from build123d import *

# Parameters (mm, degrees)
SKETCH1_W           = 20
SKETCH1_H           = 40
BOSS_EXTRUDE1_DEPTH = 20
CUT_EXTRUDE1_DEPTH  = 2


with BuildPart() as part:
    # Sketch1 → Boss-Extrude1 (new body)
    with BuildSketch(Plane(origin=(0, 0, 0), x_dir=(1, 0, 0), z_dir=(0, 1, 0))):
        Rectangle(SKETCH1_W, SKETCH1_H)
    extrude(amount=BOSS_EXTRUDE1_DEPTH)

    # Sketch2 → Cut-Extrude1 (cut)
    with BuildSketch(Plane(origin=(0, 20, 0), x_dir=(1, 0, 0), z_dir=(0, 1, 0))):
        Polygon((-3.5, -6.730769231), (-3.5, -6.416666667), (-2.064102564, -6.416666667), (-2.064102564, -4.621794872), (-3.5, -4.621794872), (-3.5, -4.307692308), (0, -4.307692308), (0, -4.621794872), (-1.705128205, -4.621794872), (-1.705128205, -6.416666667), (0, -6.416666667), (0, -6.730769231), align=None)
        Polygon((-3.5, -3.657051282), (-3.5, -3.294571314), (-2.068309295, -2.378205128), (-3.5, -1.461838942), (-3.5, -1.099358974), (-1.78505609, -2.196614583), (0, -1.054487179), (0, -1.416967147), (-1.501802885, -2.378205128), (0, -3.339443109), (0, -3.701923077), (-1.78505609, -2.559094551), align=None)
        Polygon((-3.5, -0.538461538), (-3.5, 1.615384615), (0.08974359, -0.224358974), (-0.059595353, -0.495693109), (-3.141025641, 1.083934295), (-3.141025641, -0.538461538), align=None)
        Polygon((-3.5, 2.673377404), (-3.5, 3.320512821), (0, 3.320512821), (0, 3.006410256), (-3.141025641, 3.006410256), (-3.141025641, 2.467948718), align=None)
        Polygon((-3.5, 5.365685096), (-3.5, 6.012820513), (0, 6.012820513), (0, 5.698717949), (-3.141025641, 5.698717949), (-3.141025641, 5.16025641), align=None)
    extrude(amount=-CUT_EXTRUDE1_DEPTH, mode=Mode.SUBTRACT)


solid = part.part
Check sheet for the modelled part. Datum: model origin and axes. Units: mm. A direction names the side the tool comes from. Give positions to 0.01 mm unless a question says otherwise; leave off trailing zeros. Use one line per item in the form item = value.
(1) Material ranges on line 1 along X through (y, z) = (19, 5), recorded low to high.
Answer block:
line_1 = -10 to -2.06, -1.71 to 10
(2) Tool access check on faces 1 (the flat face through (-2.79, 19.01, 2.84)), 2 (the flat face through (0, 0, 0)). Record the directions out of +Z, -Z, +X, -X, +Y, -Y that give a thin tool (end or side, any length) a straight path to the whole face; none if there is none.
Answer block:
face_1 = +Y
face_2 = +Z, -Z, +X, -X, -Y
(3) Draft check along X on faces 3 (the flat face through (-10, 10, 0)), 4 (the flat face through (-2.064, 19, 6)), 5 (the flat face through (0, 10, 20)). Enter one of: pulls with the +X half, pulls with the -X half, needs draft (parallel to the pull), parting line crosses it, or undercut.
Answer block:
face_3 = pulls with the -X half
face_4 = undercut
face_5 = needs draft
